```python
from build123d import *

# Parameters (mm, degrees)
F0_W          = 9
F0_H          = 9
F0_W_2        = 6
F0_H_2        = 6
F1_DEPTH      = 20
F2_START      = 18
F2_DEPTH      = 2
F3_R          = 1.5
F5_W          = 4
F5_H          = 4
F7_R          = 1.25
F8_DEPTH      = 25
F8_DEPTH_BACK = 25


with BuildPart() as f1:
    # F0 (on Top) → F1 (new body)
    with BuildSketch(Plane.XY):
        Rectangle(F0_W, F0_H)
        Rectangle(F0_W_2, F0_H_2, mode=Mode.SUBTRACT)
    extrude(amount=F1_DEPTH)

    # F0 (on Top) → F2 (join)
    with BuildSketch(Plane.XY.offset(F2_START)):
        Rectangle(F0_W_2, F0_H_2)
    extrude(amount=F2_DEPTH)

    # F3
    f3_edges = [f1.edges().sort_by_distance(p)[0] for p in [
        (4.5, 0, 20),
        (0, -4.5, 20),
        (-4.5, 0, 20),
        (0, 4.5, 20),
        (4.5, -4.5, 10),
        (4.5, 4.5, 10),
        (-4.5, -4.5, 10),
        (-4.5, 4.5, 10),
    ]]
    fillet(f3_edges, radius=F3_R)

    # F5 (on Right) → F6 (revolve)
    with BuildSketch(Plane.YZ):
        with Locations((0, 31.5)):
            Rectangle(F5_W, F5_H)
    revolve(axis=Axis((0, 0, 26), (0, -1, 0)))

    # F7 (on Front) → F8 (cut, two sides)
    with BuildSketch(Plane.XZ) as f8_sk:
        with Locations((0, 10)):
            Circle(F7_R)
    extrude(amount=F8_DEPTH, mode=Mode.SUBTRACT)
    extrude(f8_sk.sketch, amount=-F8_DEPTH_BACK, mode=Mode.SUBTRACT)


solid = f1.part
```
Geometry check sheet. Reference: the model listing, model coordinates, mm. A direction names the side the tool comes from. Round coordinates to 2 decimals unless told otherwise and drop trailing zeros. Loops run counter-clockwise (first coordinate to the right, second up) from the corner with the lowest first, then second, coordinate; pieces in that order, holes last. Notation, with made-up numbers: (73.25, -31.5) -> (99.25, -31.5) arc R22 ccw to (99.25, -17.5) -> close; hole circle Ø1 at (42.5, 64.25). An arc over 180 degrees is marked (long way). Use a Markdown table: item, result.
(1) Sectioned sample at D-D (z = 26). Enter the section's corners in (x, y), then the cut area to 3 significant figures.
Calculated:
| item | result |
|---|---|
| outline | (-7.5, -2) -> (-3.5, -2) -> (-3.5, 2) -> (-7.5, 2) -> close; (3.5, -2) -> (7.5, -2) -> (7.5, 2) -> (3.5, 2) -> close |
| area | 32.0 mm² |
(2) Set-up check for faces 4 (the flat face through (-3, 0, 9)), 5 (the flat face through (0, -2.5, 20)), 6 (the cylindrical face through (-0.16, -3.74, 11.24)): record each of +Z, -Z, +X, -X, +Y, -Y from which the full face is reachable in a straight line by a thin tool's end or side.
Calculated:
| item | result |
|---|---|
| face 4 | -Z |
| face 5 | +Z, +X, -X, -Y |
| face 6 | +Y, -Y |
(3) Sectioned sample at C-C (y = -0.25). Enter the section's corners in (x, z), then the cut area to 3 significant figures.
Calculated:
| item | result |
|---|---|
| outline | (-4.5, 0) -> (-3, 0) -> (-3, 18) -> (3, 18) -> (3, 0) -> (4.5, 0) -> (4.5, 18.5) arc R1.5 ccw to (3.97, 19.64) arc R7.5 ccw (long way) to (-3.97, 19.64) arc R1.5 ccw to (-4.5, 18.5) -> close; hole circle Ø7 at (0, 26) |
| area | 200 mm² |
(4) Scan lines: probe 1 along X at (y, z) = (-0.75, 26); probe 2 along X at (y, z) = (-0.75, 6); probe 3 along Y at (x, z) = (4, 28.5). Record each from-to range of solid material in increasing order.
Calculated:
| item | result |
|---|---|
| probe 1 | -7.5 to -3.5, 3.5 to 7.5 |
| probe 2 | -4.5 to -3, 3 to 4.5 |
| probe 3 | -2 to 2 |
(5) Sectioned sample at B-B (x = 0). Enter the section's corners in (y, z).
Calculated:
| item | result |
|---|---|
| outline | (-4.5, 0) -> (-3, 0) -> (-3, 8.75) -> (-4.5, 8.75) -> close; (-4.5, 11.25) -> (-3, 11.25) -> (-3, 18) -> (3, 18) -> (3, 11.25) -> (4.5, 11.25) -> (4.5, 18.5) arc R1.5 ccw to (3, 20) -> (2, 20) -> (2, 22.5) -> (-2, 22.5) -> (-2, 20) -> (-3, 20) arc R1.5 ccw to (-4.5, 18.5) -> close; (-2, 29.5) -> (2, 29.5) -> (2, 33.5) -> (-2, 33.5) -> close; (3, 0) -> (4.5, 0) -> (4.5, 8.75) -> (3, 8.75) -> close |
(6) Go/stop test with flat-tipped pins: P1, Ø1, axis at y = 0, z = 13.5, coming from the -X side; P2, Ø4, axis at y = -3, z = 22.5, coming from the -X side; P3, Ø1.8, axis at x = 0, y = -0.5, coming from the -Z side; P4, Ø2, axis at x = 4, z = 7.5, coming from the -Y side. Record where each tip stops, or that it passes through.
Calculated:
| item | result |
|---|---|
| P1 | x = -4.5 |
| P2 | x = -7.29 |
| P3 | z = 18 |
| P4 | y = -4.5 |
(7) Sectioned sample at A-A (z = 10). Enter the section's corners in (x, y), then the cut area to 3 significant figures.
Calculated:
| item | result |
|---|---|
| outline | (-4.5, -3) arc R1.5 ccw to (-3, -4.5) -> (-1.25, -4.5) -> (-1.25, -3) -> (-3, -3) -> (-3, 3) -> (-1.25, 3) -> (-1.25, 4.5) -> (-3, 4.5) arc R1.5 ccw to (-4.5, 3) -> close; (1.25, -4.5) -> (3, -4.5) arc R1.5 ccw to (4.5, -3) -> (4.5, 3) arc R1.5 ccw to (3, 4.5) -> (1.25, 4.5) -> (1.25, 3) -> (3, 3) -> (3, -3) -> (1.25, -3) -> close |
| area | 35.6 mm² |
(8) Mould release check, pull along Y, two halves, no side actions. Record for faces 1 (the flat face through (4.5, 0, 9)), 2 (the cylindrical face through (0.04, -4.07, 19.55)), 3 (the flat face through (0, 0, 18)): released by +Y, released by -Y, zero draft, split by the parting line, or undercut.
Calculated:
| item | result |
|---|---|
| face 1 | zero draft |
| face 2 | released by -Y |
| face 3 | undercut |
